from build123d import *

# Parameters (mm, degrees)
F1_DEPTH  = 5
F3_D      = 3
F4_D      = 3
F2_R      = 9.5
F2_R_2    = 6.5
F5_DEPTH  = 10
F7_DEPTH  = 8
F9_ANGLE  = 180
F10_R     = 5
F11_DEPTH = 25


with BuildPart() as f1:
    # F0 (on Top) → F1 (new body)
    with BuildSketch(Plane.XY):
        with BuildLine():
            Line((-12.5, -5), (-12.5, 5))
            Line((-12.5, 5), (-20.5, 5))
            ThreePointArc((-20.5, 5), (-21.9142135624, 4.4142135624), (-22.5, 3))
            Line((-22.5, 3), (-22.5, -3))
            ThreePointArc((-22.5, -3), (-21.9142135624, -4.4142135624), (-20.5, -5))
            Line((-20.5, -5), (-12.5, -5))
        make_face()
        with BuildLine():
            Line((0, 12.5), (-7.5, 12.5))
            ThreePointArc((-7.5, 12.5), (-11.0355339059, 11.0355339059), (-12.5, 7.5))
            Line((-12.5, 7.5), (-12.5, 5))
            Line((-12.5, 5), (-12.5, -5))
            Line((-12.5, -5), (-12.5, -7.5))
            ThreePointArc((-12.5, -7.5), (-11.0355339059, -11.0355339059), (-7.5, -12.5))
            Line((-7.5, -12.5), (0, -12.5))
            Line((0, -12.5), (7.5, -12.5))
            ThreePointArc((7.5, -12.5), (11.0355339059, -11.0355339059), (12.5, -7.5))
            Line((12.5, -7.5), (12.5, -5))
            Line((12.5, -5), (12.5, 5))
            Line((12.5, 5), (12.5, 7.5))
            ThreePointArc((12.5, 7.5), (11.0355339059, 11.0355339059), (7.5, 12.5))
            Line((7.5, 12.5), (0, 12.5))
        make_face()
        with BuildLine():
            Line((20.5, 5), (12.5, 5))
            Line((12.5, 5), (12.5, -5))
            Line((12.5, -5), (20.5, -5))
            ThreePointArc((20.5, -5), (21.9142135624, -4.4142135624), (22.5, -3))
            Line((22.5, -3), (22.5, 3))
            ThreePointArc((22.5, 3), (21.9142135624, 4.4142135624), (20.5, 5))
        make_face()
    extrude(amount=F1_DEPTH)

    # F3 (through all)
    with Locations(Plane.XY.offset(5)):
        with Locations((-17.5, 0)):
            Hole(F3_D / 2)

    # F4 (through all)
    with Locations(Plane.XY.offset(5)):
        with Locations((17.5, 0)):
            Hole(F4_D / 2)

    # F2 (on face) → F5 (join)
    with BuildSketch(Plane.XY.offset(5)):
        Circle(F2_R)
        Circle(F2_R_2, mode=Mode.SUBTRACT)
        Circle(F2_R_2)
    extrude(amount=F5_DEPTH)

    # F6 (on face) → F7 (cut)
    with BuildSketch(Plane.XY.offset(15)):
        with BuildLine():
            ThreePointArc((-4.8296291314, -1.2940952255), (-5, 0), (-4.8296291314, 1.2940952255))
            Line((-4.8296291314, 1.2940952255), (-9.1762953497, 2.4587809285))
            ThreePointArc((-9.1762953497, 2.4587809285), (-9.5, 0), (-9.1762953497, -2.4587809285))
            Line((-9.1762953497, -2.4587809285), (-4.8296291314, -1.2940952255))
        make_face()
        with BuildLine():
            Line((1.2940952255, -4.8296291314), (2.4587809285, -9.1762953497))
            ThreePointArc((2.4587809285, -9.1762953497), (4.75, -8.227241336), (6.7175144213, -6.7175144213))
            Line((6.7175144213, -6.7175144213), (3.5355339059, -3.5355339059))
            ThreePointArc((3.5355339059, -3.5355339059), (2.5, -4.3301270189), (1.2940952255, -4.8296291314))
        make_face()
        with BuildLine():
            Line((3.5355339059, 3.5355339059), (6.7175144213, 6.7175144213))
            ThreePointArc((6.7175144213, 6.7175144213), (4.75, 8.227241336), (2.4587809285, 9.1762953497))
            Line((2.4587809285, 9.1762953497), (1.2940952255, 4.8296291314))
            ThreePointArc((1.2940952255, 4.8296291314), (2.5, 4.3301270189), (3.5355339059, 3.5355339059))
        make_face()
    extrude(amount=-F7_DEPTH, mode=Mode.SUBTRACT)

    # F8 (on face) → F9 (revolve, cut)
    with BuildSketch(Plane.XY.offset(15)):
        with BuildLine():
            Line((-6.5, 0), (-5, 0))
            ThreePointArc((-5, 0), (-4.9572243069, 0.6526309611), (-4.8296291314, 1.2940952255))
            Line((-4.8296291314, 1.2940952255), (-6.2785178709, 1.6823237932))
            ThreePointArc((-6.2785178709, 1.6823237932), (-6.4443915989, 0.8484202494), (-6.5, 0))
        make_face()
        with BuildLine():
            Line((-5, 0), (6.5, 0))
            ThreePointArc((6.5, 0), (6.0052169613, 2.4874423104), (4.5961940777, 4.5961940777))
            Line((4.5961940777, 4.5961940777), (3.5355339059, 3.5355339059))
            ThreePointArc((3.5355339059, 3.5355339059), (2.5, 4.3301270189), (1.2940952255, 4.8296291314))
            Line((1.2940952255, 4.8296291314), (1.6823237932, 6.2785178709))
            ThreePointArc((1.6823237932, 6.2785178709), (-3.25, 5.6291651246), (-6.2785178709, 1.6823237932))
            Line((-6.2785178709, 1.6823237932), (-4.8296291314, 1.2940952255))
            ThreePointArc((-4.8296291314, 1.2940952255), (-4.9572243069, 0.6526309611), (-5, 0))
        make_face()
        with BuildLine():
            Line((3.5355339059, 3.5355339059), (4.5961940777, 4.5961940777))
            ThreePointArc((4.5961940777, 4.5961940777), (3.25, 5.6291651246), (1.6823237932, 6.2785178709))
            Line((1.6823237932, 6.2785178709), (1.2940952255, 4.8296291314))
            ThreePointArc((1.2940952255, 4.8296291314), (2.5, 4.3301270189), (3.5355339059, 3.5355339059))
        make_face()
    revolve(axis=Axis((0, 0, 15), (-1, 0, 0)), revolution_arc=F9_ANGLE, mode=Mode.SUBTRACT)

    # F10 (on face) → F11 (cut)
    with BuildSketch(Plane(origin=(0, 0, 0), x_dir=(1, 0, 0), z_dir=(0, 0, -1))):
        Circle(F10_R)
    extrude(amount=-F11_DEPTH, mode=Mode.SUBTRACT)


solid = f1.part
Geometry check sheet. Reference: the model listing, model coordinates, mm. A direction names the side the tool comes from. Give positions to 0.01 mm unless a question says otherwise; leave off trailing zeros. Write each loop counter-clockwise with the first axis right and the second up, starting at its lowest first coordinate (ties: lowest second). Pieces come first, ordered by that corner, then holes.
1) Cross-section at B-B (y = 0). Record the boundary of the cut face in (x, z), plus the area to 3 significant figures.
Values follow:
outline: (-22.5, 0) - (-19, 0) - (-19, 5) - (-22.5, 5) - close; (-16, 0) - (-5, 0) - (-5, 7) - (-9.5, 7) - (-9.5, 5) - (-16, 5) - close; (5, 0) - (16, 0) - (16, 5) - (9.5, 5) - (9.5, 15) - (6.5, 15) arc R6.5 cw to (5, 10.85) - close; (19, 0) - (22.5, 0) - (22.5, 5) - (19, 5) - close
area: 195 mm2
2) Go/stop test with flat-tipped pins: pin 1 Ø3.5 at (x, y) = (17.5, 0) entering from -Z; pin 2 Ø0.8 at (y, z) = (6.5, 2) entering from +X; pin 3 Ø5.5 at (x, z) = (-18, 1.5) entering from +Y; pin 4 Ø2 at (x, y) = (8.5, 7.5) entering from +Z. Record where each tip stops, or that it passes through.
Values follow:
pin 1: stops at z = 0
pin 2: stops at x = 12.5
pin 3: stops at y = 5
pin 4: stops at z = 5
3) Release check for a two-part mould opening along Y. For faces 1 (the face through (11, -11.07, 2.46)), 2 (the face through (-12.5, 6, 2)), 3 (the face through (-6.973, 1.868, 11.056)) record: released by +Y, released by -Y, zero draft, split by the parting line, or undercut.
Values follow:
face 1: released by -Y
face 2: zero draft
face 3: undercut
4) Cross-section at A-A (z = 1.5). Record the boundary of the cut face in (x, y), plus the area to 3 significant figures.
Values follow:
outline: (-22.5, -3) arc R2 ccw to (-20.5, -5) - (-12.5, -5) - (-12.5, -7.5) arc R5 ccw to (-7.5, -12.5) - (7.5, -12.5) arc R5 ccw to (12.5, -7.5) - (12.5, -5) - (20.5, -5) arc R2 ccw to (22.5, -3) - (22.5, 3) arc R2 ccw to (20.5, 5) - (12.5, 5) - (12.5, 7.5) arc R5 ccw to (7.5, 12.5) - (-7.5, 12.5) arc R5 ccw to (-12.5, 7.5) - (-12.5, 5) - (-20.5, 5) arc R2 ccw to (-22.5, 3) - close; hole circle Ø3 at (-17.5, 0); hole circle Ø10 at (0, 0); hole circle Ø3 at (17.5, 0)
area: 707 mm2
5) Cross-section at C-C (x = -17.5). Record the boundary of the cut face in (y, z), plus the area to 3 significant figures.
Values follow:
outline: (-5, 0) - (-1.5, 0) - (-1.5, 5) - (-5, 5) - close; (1.5, 0) - (5, 0) - (5, 5) - (1.5, 5) - close
area: 35.0 mm2
6) Set-up check for faces 4 (the face through (-16, 5, 2)), 5 (the face through (1.868, -6.973, 11.056)), 6 (the face through (-7.033, -1.885, 11.056)), 7 (the face through (12.5, -6, 2)), 8 (the face through (5, 5, 11)): record each of +Z, -Z, +X, -X, +Y, -Y from which the full face is reachable in a straight line by a thin tool's end or side.
Values follow:
face 4: +Z, -Z, -X, +Y
face 5: +Z
face 6: +Z, -X
face 7: +Z, -Z, +X, -Y
face 8: +Z, +Y
7) Thickness scan on line 1 (Y direction, x = 0, z = 6.25); line 2 (Y direction, x = -17.5, z = 3.7); line 3 (Z direction, x = -15.5, y = 0.75). Record the ranges inside material, lowest first.
Values follow:
line 1: y = -9.5 to -5, 5 to 9.5
line 2: y = -5 to -1.5, 1.5 to 5
line 3: z = 0 to 5
8) Cross-section at D-D (z = 13.5). Record the boundary of the cut face in (x, y), plus the area to 3 significant figures.
Values follow:
outline: (-9.18, -2.46) arc R9.5 ccw to (2.46, -9.18) - (1.64, -6.11) arc R6.32 cw to (-6.11, -1.64) - close; (-9.18, 2.46) - (-6.11, 1.64) arc R6.32 cw to (1.64, 6.11) - (2.46, 9.18) arc R9.5 ccw to start; (4.47, -4.47) - (6.72, -6.72) arc R9.5 ccw to (6.72, 6.72) - (4.47, 4.47) arc R6.32 cw to start
area: 118 mm2
